Source: CAD feature listing. Evaluate the final solid. Frame: model axes, mm. Face numbers are marked on the shaded views. A direction names the side the tool comes from. Give positions to 0.01 mm unless a question says otherwise; leave off trailing zeros. Order: outer loops, then holes, each group sorted by start corner. A loop starts at its lowest first (then second) coordinate and runs counter-clockwise, first axis right, second up. Notation, with made-up numbers: (64.25, 11) - (76.25, 11) arc R15 cw to (76.25, 36) - close; hole circle Ø6 at (19.25, 68). An arc over 180 degrees is marked (long way). Write each question's results on one line, items separated by ' | '. Start each with the question number.
Item 1: Section B-B on x = 37. Output: boundary loops of the cut face in (y, z), and give its area (3 significant figures).
Item 2: Mould query, pull axis Y, two halves, no side actions, for the marked faces 1, 2 and 3. Classes: released by +Y, released by -Y, zero draft, split by the parting line, or undercut.
Item 3: Line query: line 1 along Y through (x, z) = (-49, 6.25); line 2 along Y through (x, z) = (-45, 5); line 3 along X through (y, z) = (-52.5, 5.25). Output: solid intervals per line, ascending.
Item 4: Set-up query: the marked faces 4, 5 and 6. Return all of +Z, -Z, +X, -X, +Y, -Y with unobstructed straight access to the full face (end or side cutting, diameter ignored); none if empty.
Item 5: Section C-C on y = 11.5. Output: boundary loops of the cut face in (x, z), and give its area (3 significant figures).
Item 6: Section D-D on x = -41.5. Output: boundary loops of the cut face in (y, z), and give its area (3 significant figures).
Item 7: Contact query for flat-ended pins moving along their axis: pin 1 Ø5 at (y, z) = (10.5, 2) entering from +X; pin 2 Ø4 at (x, z) = (39.5, 6) entering from -Y; pin 3 Ø2.5 at (y, z) = (-59.5, 4) entering from +X; pin 4 Ø1.5 at (x, z) = (-15.5, 8) entering from -Y. Output: stop coordinate, or through.
```python
from build123d import *

# Parameters (mm, degrees)
F1_DEPTH    = 9.144
F2_T1_DEPTH = 18.034


# Not quite as in the source:
# - a fillet or chamfer that OpenCascade refuses, or shapes differently, is made with other operations: its cross-section is extruded or revolved along the edge and cut away or added


with BuildPart() as f1:
    # F0 (on Top) → F1 (new body)
    with BuildSketch(Plane.XY):
        Polygon((-45.8869487338, 19.8141042413), (-45.8869487338, 21.5921042413), (-54.2689487338, 21.5921042413), (-54.2689487338, 12.9561042413), (-49.1889487338, 12.9561042413), (-49.1889487338, -61.4658957587), (-37.2509487338, -61.4658957587), (-37.2509487338, -56.6398957587), (-40.0449487338, -56.6398957587), (-40.0449487338, -58.6718957587), (-46.3949487338, -58.6718957587), (-46.3949487338, -37.378154695), (-46.3949487338, -27.9378957587), (-46.3949487338, -24.8898957587), (-40.0449487338, -24.8898957587), (-40.0449487338, -26.9218957587), (-37.2509487338, -26.9218957587), (-37.2509487338, -22.0958957587), (-46.3949487338, -22.0958957587), (-7.7869487338, 12.9561042413), (44.2830512662, 12.9561042413), (44.2830512662, 21.5921042413), (35.9010512662, 21.5921042413), (35.9010512662, 19.8141042413), (40.7270512662, 19.8141042413), (40.7270512662, 16.0041042413), (-50.7129487338, 16.0041042413), (-50.7129487338, 19.8141042413), align=None)
        Polygon((-11.7646907362, 12.9561042413), (-46.3949487338, -18.4845247302), (-46.3949487338, 12.9561042413), align=None, mode=Mode.SUBTRACT)
    extrude(amount=F1_DEPTH)

    # F2: fillet of radius 1.778 on 4 edges, made by hand

    # F2_s2 → F2_t1 (cut)
    with BuildSketch(Plane.XY.offset(-4.445)):
        with BuildLine():
            ThreePointArc((-38.2669487338, -26.9218957587), (-39.5241845908, -26.4011316156), (-40.0449487338, -25.1438957587))
            Line((-40.0449487338, -25.1438957587), (-40.0449487338, -26.9218957587))
            Line((-40.0449487338, -26.9218957587), (-38.2669487338, -26.9218957587))
        make_face()
        with BuildLine():
            ThreePointArc((-37.2509487338, -25.1438957587), (-37.7717128769, -26.4011316156), (-39.0289487338, -26.9218957587))
            Line((-39.0289487338, -26.9218957587), (-37.2509487338, -26.9218957587))
            Line((-37.2509487338, -26.9218957587), (-37.2509487338, -25.1438957587))
        make_face()
        with BuildLine():
            ThreePointArc((-39.0289487338, -56.6398957587), (-37.7717128769, -57.1606599017), (-37.2509487338, -58.4178957587))
            Line((-37.2509487338, -58.4178957587), (-37.2509487338, -56.6398957587))
            Line((-37.2509487338, -56.6398957587), (-39.0289487338, -56.6398957587))
        make_face()
        with BuildLine():
            ThreePointArc((-40.0449487338, -58.4178957587), (-39.5241845908, -57.1606599017), (-38.2669487338, -56.6398957587))
            Line((-38.2669487338, -56.6398957587), (-40.0449487338, -56.6398957587))
            Line((-40.0449487338, -56.6398957587), (-40.0449487338, -58.4178957587))
        make_face()
    extrude(amount=F2_T1_DEPTH, mode=Mode.SUBTRACT)


solid = f1.part
```
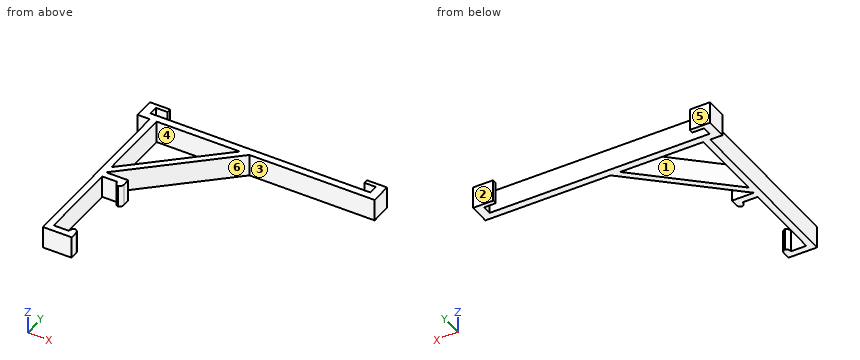
Evaluation:
1) outline: (12.96, 0) - (16, 0) - (16, 9.14) - (12.96, 9.14) - close; (19.81, 0) - (21.59, 0) - (21.59, 9.14) - (19.81, 9.14) - close | area: 44.1 mm^2
2) face 1: undercut | face 2: released by +Y | face 3: released by -Y
3) line 1: y = -61.47 to 16, 19.81 to 21.59 | line 2: y = -61.47 to -58.67, -24.89 to -22.1, -20.83 to -17.22, 12.96 to 16 | line 3: x = -49.19 to -46.39
4) face 4: +Z, -Z | face 5: +Z, -Z, +X, -X, +Y | face 6: +Z, -Z, +X
5) outline: (-49.19, 0) - (-46.39, 0) - (-46.39, 9.14) - (-49.19, 9.14) - close; (-13.37, 0) - (-9.39, 0) - (-9.39, 9.14) - (-13.37, 9.14) - close | area: 61.9 mm^2
6) outline: (-61.47, 0) - (-58.67, 0) - (-58.67, 9.14) - (-61.47, 9.14) - close; (-24.89, 0) - (-22.1, 0) - (-22.1, 9.14) - (-24.89, 9.14) - close; (-17.65, 0) - (-14.04, 0) - (-14.04, 9.14) - (-17.65, 9.14) - close; (12.96, 0) - (16, 0) - (16, 9.14) - (12.96, 9.14) - close | area: 112 mm^2
7) pin 1: stops at x = 44.28 | pin 2: stops at y = 12.96 | pin 3: stops at x = -37.25 | pin 4: stops at y = 5.27
